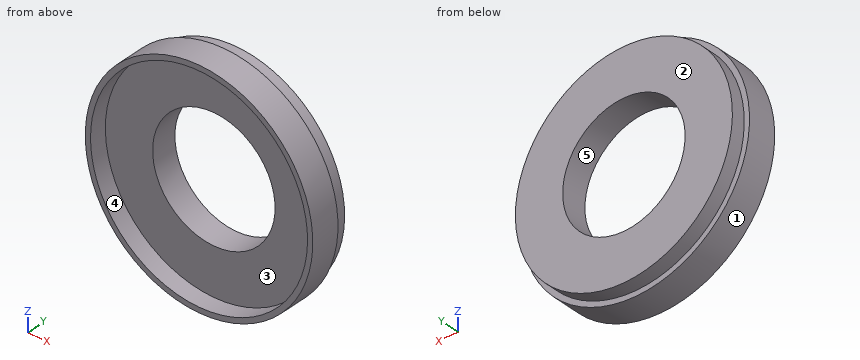
```python
from build123d import *

# Parameters (mm, degrees)
SZKIC1_W = 3
SZKIC1_H = 10


with BuildPart() as part:
    # Szkic1 → Obrót1 (revolve)
    with BuildSketch(Plane.XY, mode=Mode.PRIVATE) as obr_t1_sk:
        Polygon((-62, 0), (-35, 0), (-35, 15), (-62, 15), (-62, 7), (-65, 7), (-65, 0), align=None)
        with Locations((-63.5, -5)):
            Rectangle(SZKIC1_W, SZKIC1_H)
    revolve(obr_t1_sk.sketch.rotate(Axis((0, 0, 0), (0, 1, 0)), 270), axis=Axis((0, 0, 0), (0, 1, 0)))


solid = part.part
```
Geometry: final body of the model. Coordinates: model frame, mm. Face numbers are marked on the shaded views. A direction names the side the tool comes from. Round coordinates to 2 decimals unless told otherwise and drop trailing zeros. Loops run counter-clockwise (first coordinate to the right, second up) from the corner with the lowest first, then second, coordinate; pieces in that order, holes last. Notation, with made-up numbers: (54.5, 87.5) -> (88.5, 87.5) arc R13 ccw to (88.5, 103.5) -> close; hole circle Ø8 at (81, -9). An arc over 180 degrees is marked (long way). Use one line per item in the form item = value. Start each with the question number.
1) Section C-C on y = -4.75. Output: boundary loops of the cut face in (x, z).
2) Section B-B on x = 0. Output: boundary loops of the cut face in (y, z).
3) Section A-A on z = 0. Output: boundary loops of the cut face in (x, y).
4) First-contact query: P1, Ø5, axis at y = -2.5, z = -14.5, coming from the +X side; P2, Ø1, axis at x = 5, y = 4.5, coming from the +Z side; P3, Ø5, axis at x = 48, y = 11, coming from the -Z side. Flat tips, straight axial feed; report the tip coordinate or a pass-through.
5) Section D-D on z = 49.5. Output: boundary loops of the cut face in (x, y).
6) Draft query along X for the marked faces 1, 2 and 3. Return one class per face: released by +X, released by -X, zero draft, split by the parting line, or undercut.
7) Access query for the marked faces 4 and 5. Directions: +Z, -Z, +X, -X, +Y, -Y. A direction counts if a zero-diameter tool reaches every point of the face in a straight line with its end or side. Return the directions, or none.
8) Line query: L1, parallel to X at y = -8, z = 0; L2, parallel to X at y = 4, z = 0; L3, parallel to Y at x = 10, z = 47.5. Output: solid intervals per line, ascending.
Response:
q1.outline = circle Ø130 at (0, 0); hole circle Ø124 at (0, 0)
q2.outline = (-10, -65) -> (7, -65) -> (7, -62) -> (15, -62) -> (15, -35) -> (0, -35) -> (0, -62) -> (-10, -62) -> close; (-10, 62) -> (0, 62) -> (0, 35) -> (15, 35) -> (15, 62) -> (7, 62) -> (7, 65) -> (-10, 65) -> close
q3.outline = (-65, -10) -> (-62, -10) -> (-62, 0) -> (-35, 0) -> (-35, 15) -> (-62, 15) -> (-62, 7) -> (-65, 7) -> close; (35, 0) -> (62, 0) -> (62, -10) -> (65, -10) -> (65, 7) -> (62, 7) -> (62, 15) -> (35, 15) -> close
q4.P1 = 63.88
q4.P2 = 64.84
q4.P3 = -42.12
q5.outline = (-42.13, -10) -> (-37.33, -10) -> (-37.33, 0) -> (37.33, 0) -> (37.33, -10) -> (42.13, -10) -> (42.13, 7) -> (37.33, 7) -> (37.33, 15) -> (-37.33, 15) -> (-37.33, 7) -> (-42.13, 7) -> close
q6.face_1 = split by the parting line
q6.face_2 = zero draft
q6.face_3 = undercut
q7.face_4 = -Y
q7.face_5 = +Y, -Y
q8.L1 = -65 to -62, 62 to 65
q8.L2 = -65 to -35, 35 to 65
q8.L3 = 0 to 15
